```python
from build123d import *

# Parameters (mm, degrees)
EXTRUDE_1_DEPTH     = 4
SKETCH_2_R          = 1.525
CUT_EXTRUDE_1_DEPTH = 5
SKETCH_4_R          = 10
CUT_EXTRUDE_2_DEPTH = 5
SKETCH_7_R          = 18.75
CUT_EXTRUDE_4_DEPTH = 5
SKETCH_8_R          = 1.525
CUT_EXTRUDE_5_DEPTH = 5
SKETCH_9_R          = 1.525
CUT_EXTRUDE_6_DEPTH = 5
FILLET_1_R          = 2
CUT_EXTRUDE_8_DEPTH = 5
FILLET_2_R          = 2


with BuildPart() as part:
    # 草图1 → 凸台-拉伸1 (new body)
    with BuildSketch(Plane(origin=(0, 0, 0), x_dir=(1, 0, 0), z_dir=(0, 1, 0))):
        with BuildLine():
            ThreePointArc((-32.25, 28.5), (-60.75, 0), (-32.25, -28.5))
            Line((-32.25, -28.5), (-32.25, 28.5))
        make_face()
        with BuildLine():
            Line((-32.25, 28.5), (-32.25, -28.5))
            ThreePointArc((-32.25, -28.5), (-12.097456736, -20.152543264), (-3.75, 0))
            ThreePointArc((-3.75, 0), (-12.097456736, 20.152543264), (-32.25, 28.5))
        make_face()
        with BuildLine():
            ThreePointArc((-3.75, 0), (-12.097456736, -20.152543264), (-32.25, -28.5))
            Line((-32.25, -28.5), (32.25, -28.5))
            Line((32.25, -28.5), (32.25, 28.5))
            Line((32.25, 28.5), (-32.25, 28.5))
            ThreePointArc((-32.25, 28.5), (-12.097456736, 20.152543264), (-3.75, 0))
        make_face()
    extrude(amount=EXTRUDE_1_DEPTH)

    # 草图2 → 切除-拉伸1 (cut, through all)
    with BuildSketch(Plane(origin=(0, 4, 0), x_dir=(1, 0, 0), z_dir=(0, 1, 0))):
        with Locations((-45.75, 0)):
            Circle(SKETCH_2_R)
        with Locations((-39, 11.691342951)):
            Circle(SKETCH_2_R)
        with Locations((-25.5, 11.691342951)):
            Circle(SKETCH_2_R)
        with Locations((-18.75, 0)):
            Circle(SKETCH_2_R)
        with Locations((-25.5, -11.691342951)):
            Circle(SKETCH_2_R)
        with Locations((-39, -11.691342951)):
            Circle(SKETCH_2_R)
    extrude(amount=-CUT_EXTRUDE_1_DEPTH, mode=Mode.SUBTRACT)

    # 草图4 → 切除-拉伸2 (cut, through all)
    with BuildSketch(Plane(origin=(0, 4, 0), x_dir=(1, 0, 0), z_dir=(0, 1, 0))):
        with Locations((-32.25, 0)):
            Circle(SKETCH_4_R)
    extrude(amount=-CUT_EXTRUDE_2_DEPTH, mode=Mode.SUBTRACT)

    # 草图7 → 切除-拉伸4 (cut, through all)
    with BuildSketch(Plane(origin=(0, 4, 0), x_dir=(1, 0, 0), z_dir=(0, 1, 0))):
        with Locations((-32.25, 0)):
            Circle(SKETCH_7_R)
    extrude(amount=-CUT_EXTRUDE_4_DEPTH, mode=Mode.SUBTRACT)

    # 草图8 → 切除-拉伸5 (cut, through all)
    with BuildSketch(Plane(origin=(0, 4, 0), x_dir=(1, 0, 0), z_dir=(0, 1, 0))):
        with Locations((-32.25, 25)):
            Circle(SKETCH_8_R)
        with Locations((-19.75, 21.650635095)):
            Circle(SKETCH_8_R)
        with Locations((-10.599364905, 12.5)):
            Circle(SKETCH_8_R)
        with Locations((-7.25, 0)):
            Circle(SKETCH_8_R)
        with Locations((-10.599364905, -12.5)):
            Circle(SKETCH_8_R)
        with Locations((-19.75, -21.650635095)):
            Circle(SKETCH_8_R)
        with Locations((-32.25, -25)):
            Circle(SKETCH_8_R)
        with Locations((-44.75, -21.650635095)):
            Circle(SKETCH_8_R)
        with Locations((-53.900635095, -12.5)):
            Circle(SKETCH_8_R)
        with Locations((-57.25, 0)):
            Circle(SKETCH_8_R)
        with Locations((-53.900635095, 12.5)):
            Circle(SKETCH_8_R)
        with Locations((-44.75, 21.650635095)):
            Circle(SKETCH_8_R)
    extrude(amount=-CUT_EXTRUDE_5_DEPTH, mode=Mode.SUBTRACT)

    # 草图9 → 切除-拉伸6 (cut, through all)
    with BuildSketch(Plane(origin=(0, 4, 0), x_dir=(1, 0, 0), z_dir=(0, 1, 0))):
        with Locations((29.25, 0)):
            Circle(SKETCH_9_R)
        with Locations((29.25, 20)):
            Circle(SKETCH_9_R)
        with Locations((29.25, -20)):
            Circle(SKETCH_9_R)
    extrude(amount=-CUT_EXTRUDE_6_DEPTH, mode=Mode.SUBTRACT)

    # 圆角1
    fillet_1_edges = [part.edges().sort_by_distance(p)[0] for p in [
        (32.25, 2, -28.5),
        (32.25, 2, 28.5),
    ]]
    fillet(fillet_1_edges, radius=FILLET_1_R)

    # 草图18 → 切除-拉伸8 (cut, through all)
    with BuildSketch(Plane(origin=(0, 4, 0), x_dir=(1, 0, 0), z_dir=(0, 1, 0))):
        with BuildLine():
            Line((18.25, 22.5), (-5.440486763, 22.5))
            ThreePointArc((-5.440486763, 22.5), (-0.100467085, 13.835011143), (2.520677301, 4))
            Line((2.520677301, 4), (18.25, 4))
            Line((18.25, 4), (18.25, 22.5))
        make_face()
        with BuildLine():
            Line((-5.440486763, -22.5), (18.25, -22.5))
            Line((18.25, -22.5), (18.25, -3))
            Line((18.25, -3), (2.621191548, -3))
            ThreePointArc((2.621191548, -3), (0.094857948, -13.371991785), (-5.440486763, -22.5))
        make_face()
    extrude(amount=-CUT_EXTRUDE_8_DEPTH, mode=Mode.SUBTRACT)

    # 圆角2
    fillet_2_edges = [part.edges().sort_by_distance(p)[0] for p in [
        (2.520677301, 2, -4),
        (-5.440486763, 2, -22.5),
        (18.25, 2, -22.5),
        (18.25, 2, -4),
        (-5.440486763, 2, 22.5),
        (2.621191548, 2, 3),
        (18.25, 2, 3),
        (18.25, 2, 22.5),
    ]]
    fillet(fillet_2_edges, radius=FILLET_2_R)


solid = part.part
```
Geometry: final body of the model. Coordinates: model frame, mm. A direction names the side the tool comes from. Round coordinates to 2 decimals unless told otherwise and drop trailing zeros. Loops run counter-clockwise (first coordinate to the right, second up) from the corner with the lowest first, then second, coordinate; pieces in that order, holes last. Notation, with made-up numbers: (41.5, -20) -> (78.5, -20) arc R20 ccw to (78.5, 10) -> close; hole circle Ø9 at (62, 71). An arc over 180 degrees is marked (long way). Write each question's results on one line, items separated by ' | '.
Item 1: Cut plane D-D on z = 25. Return the cut outline in (x, y) (3 decimals), and give its area (3 significant figures).
Answers below:
outline: (-45.934, 0) -> (-33.775, 0) -> (-33.775, 4) -> (-45.934, 4) -> close; (-30.725, 0) -> (32.25, 0) -> (32.25, 4) -> (-30.725, 4) -> close | area: 301 mm²
Item 2: Pull-direction query (Z, two-part tool) for faces 3 (the face through (-33.46, 2.03, -24.07)), 4 (the face through (-60.743, 1.972, -0.627)), 5 (the face through (31.65, 2.03, 27.93)), 6 (the face through (-33.46, 2.03, 25.93)); classes: pulls with the +Z half, pulls with the -Z half, needs draft (parallel to the pull), parting line crosses it, or undercut.
Answers below:
face 3: undercut | face 4: parting line crosses it | face 5: pulls with the +Z half | face 6: undercut
Item 3: Set-up query: faces 1 (the face through (-3.197, 1.972, -21.471)), 2 (the face through (-1, 2, -28.5)). Return all of +Z, -Z, +X, -X, +Y, -Y with unobstructed straight access to the full face (end or side cutting, diameter ignored); none if empty.
Answers below:
face 1: +Y, -Y | face 2: -Z, +X, -X, +Y, -Y
Item 4: Line query: probe 1 along Z at (x, y) = (13.5, 3.65); probe 2 along Z at (x, y) = (-32.25, 1.8) (3 decimals); probe 3 along X at (y, z) = (2, 20) (3 decimals). Output: solid intervals per line, ascending. Write a range as [from, to].
Answers below:
probe 1: z = [-28.5, -22.5], [-4, 3], [22.5, 28.5] | probe 2: z = [-28.5, -26.525], [-23.475, -18.75], [18.75, 23.475], [26.525, 28.5] | probe 3: x = [-52.554, -3.385], [18.25, 27.725], [30.775, 32.25]
Item 5: Cut plane A-A on x = 9.5. Return the cut outline in (y, z).
Answers below:
outline: (0, -28.5) -> (4, -28.5) -> (4, -22.5) -> (0, -22.5) -> close; (0, -4) -> (4, -4) -> (4, 3) -> (0, 3) -> close; (0, 22.5) -> (4, 22.5) -> (4, 28.5) -> (0, 28.5) -> close
Item 6: Pin query (flat end, axial travel): pin 1 Ø2.5 at (x, z) = (-7.25, 0) entering from +Y; pin 2 Ø3.5 at (x, z) = (-32.25, -25) entering from +Y; pin 3 Ø2 at (x, y) = (-47, 3) entering from -Z; pin 4 Ø1 at (x, y) = (-37, 2) entering from +Z. Return the tip coordinate at first contact, or that it passes through.
Answers below:
pin 1: passes through | pin 2: stops at y = 4 | pin 3: stops at z = -24.96 | pin 4: stops at z = 28.18
Item 7: Cut plane B-B on z = 0. Return the cut outline in (x, y) (3 decimals).
Answers below:
outline: (-60.75, 0) -> (-58.775, 0) -> (-58.775, 4) -> (-60.75, 4) -> close; (-55.725, 0) -> (-51, 0) -> (-51, 4) -> (-55.725, 4) -> close; (-13.5, 0) -> (-8.775, 0) -> (-8.775, 4) -> (-13.5, 4) -> close; (-5.725, 0) -> (27.725, 0) -> (27.725, 4) -> (-5.725, 4) -> close; (30.775, 0) -> (32.25, 0) -> (32.25, 4) -> (30.775, 4) -> close
Item 8: Cut plane C-C on x = -7.25. Return the cut outline in (y, z) (3 decimals).
Answers below:
outline: (0, -28.5) -> (4, -28.5) -> (4, -1.525) -> (0, -1.525) -> close; (0, 1.525) -> (4, 1.525) -> (4, 28.5) -> (0, 28.5) -> close
